from build123d import *

# Parameters (mm, degrees)
SKETCH1_R           = 50
SKETCH1_R_2         = 4
BOSS_EXTRUDE1_DEPTH = 10
BOSS_EXTRUDE2_START = 50
SKETCH2_R           = 50
SKETCH2_R_2         = 40
BOSS_EXTRUDE2_DEPTH = 50
BOSS_EXTRUDE3_START = 10
SKETCH4_R           = 4
SKETCH4_R_2         = 40
BOSS_EXTRUDE3_DEPTH = 10


with BuildPart() as part:
    # Sketch1 → Boss-Extrude1 (new body)
    with BuildSketch(Plane(origin=(0, 0, 0), x_dir=(1, 0, 0), z_dir=(0, 1, 0))):
        with Locations(Location((0, 0, 0), (0, 0, 270))):
            Circle(SKETCH1_R)
        with Locations(Location((0, 0, 0), (0, 0, 270))):
            Circle(SKETCH1_R_2, mode=Mode.SUBTRACT)
    extrude(amount=BOSS_EXTRUDE1_DEPTH)

    # Sketch2 → Boss-Extrude2 (add)
    with BuildSketch(Plane.XZ.offset(BOSS_EXTRUDE2_START)):
        with Locations(Location((0, 0, 0), (0, 0, 270))):
            Circle(SKETCH2_R)
        with Locations(Location((0, 0, 0), (0, 0, 270))):
            Circle(SKETCH2_R_2, mode=Mode.SUBTRACT)
    extrude(amount=-BOSS_EXTRUDE2_DEPTH)

    # Sketch4 → Boss-Extrude3 (add)
    with BuildSketch(Plane.XZ.offset(50).offset(BOSS_EXTRUDE3_START)):
        with BuildLine():
            Line((-30.18665216, -50), (29.99743133, -50))
            Line((29.99743133, -50), (45.000642085, -58.660624714))
            ThreePointArc((45.000642085, -58.660624714), (57.090562914, -57.051518812), (58.632887989, -44.95289737))
            Line((58.632887989, -44.95289737), (50, -30.18665216))
            Line((50, -30.18665216), (50, 29.99743133))
            Line((50, 29.99743133), (58.660624714, 45.000642085))
            ThreePointArc((58.660624714, 45.000642085), (57.051518812, 57.090562914), (44.95289737, 58.632887989))
            Line((44.95289737, 58.632887989), (30.18665216, 50))
            Line((30.18665216, 50), (-29.99743133, 50))
            Line((-29.99743133, 50), (-45.000642085, 58.660624714))
            ThreePointArc((-45.000642085, 58.660624714), (-57.090562914, 57.051518812), (-58.632887989, 44.95289737))
            Line((-58.632887989, 44.95289737), (-50, 30.18665216))
            Line((-50, 30.18665216), (-50, -29.99743133))
            Line((-50, -29.99743133), (-58.660624714, -45.000642085))
            ThreePointArc((-58.660624714, -45.000642085), (-57.051518812, -57.090562914), (-44.95289737, -58.632887989))
            Line((-44.95289737, -58.632887989), (-30.18665216, -50))
        make_face()
        with Locations(Location((-50, 50, 0), (0, 0, 270))):
            Circle(SKETCH4_R, mode=Mode.SUBTRACT)
        with Locations(Location((-50, -50, 0), (0, 0, 270))):
            Circle(SKETCH4_R, mode=Mode.SUBTRACT)
        with Locations(Location((50, -50, 0), (0, 0, 90))):
            Circle(SKETCH4_R, mode=Mode.SUBTRACT)
        with Locations(Location((50, 50, 0), (0, 0, 90))):
            Circle(SKETCH4_R, mode=Mode.SUBTRACT)
        with Locations(Location((0, 0, 0), (0, 0, 270))):
            Circle(SKETCH4_R_2, mode=Mode.SUBTRACT)
    extrude(amount=-BOSS_EXTRUDE3_DEPTH)


solid = part.part
The listing builds one solid part. Answer for the finished solid, in the listing's coordinates (mm). A direction names the side the tool comes from. Give positions to 0.01 mm unless a question says otherwise; leave off trailing zeros. Write each loop counter-clockwise with the first axis right and the second up, starting at its lowest first coordinate (ties: lowest second). Pieces come first, ordered by that corner, then holes. Notation, with made-up numbers: (-29, -26.75) -> (4, -26.75) arc R17 ccw to (4, -0.75) -> close; hole circle Ø11 at (55.5, 12). An arc over 180 degrees is marked (long way). Use a Markdown table: item, result.
(1) Section D-D, the plane z = 48 is taken. Determine the outline of the cut face in (x, y).
Return value:
| item | result |
|---|---|
| outline | (-59.8, -60) -> (-53.46, -60) -> (-53.46, -50) -> (-59.8, -50) -> close; (-46.54, -60) -> (46.54, -60) -> (46.54, -50) -> (14, -50) -> (14, 10) -> (-14, 10) -> (-14, -50) -> (-46.54, -50) -> close; (53.46, -60) -> (59.8, -60) -> (59.8, -50) -> (53.46, -50) -> close |
(2) Section A-A, the plane y = -1.5 is taken. Determine the outline of the cut face in (x, z).
Return value:
| item | result |
|---|---|
| outline | circle Ø100 at (0, 0); hole circle Ø80 at (0, 0) |
(3) For faces 4 (the flat face through (54.27, -55.07, 37.394)), 5 (the flat face through (1, 0, 8)), 6 (the flat face through (-50, -55, 1)), 7 (the flat face through (-37.394, -55.07, 54.27)), 8 (the flat face through (-1, -55, -50)), determine the directions among +Z, -Z, +X, -X, +Y, -Y from which every point of the face is accessible in a straight line to the end or side of a thin tool.
Return value:
| item | result |
|---|---|
| face 4 | +X, +Y, -Y |
| face 5 | -Y |
| face 6 | -X, +Y, -Y |
| face 7 | +Z, +Y, -Y |
| face 8 | -Z, +Y, -Y |
(4) Determine the mould class of faces 1 (the flat face through (37.673, -55.07, 54.377)), 2 (the cylindrical face through (-52.4, -55.1, 53.2)), 3 (the flat face through (-41, -50, 43)) for opening direction Z: released by +Z, released by -Z, zero draft, split by the parting line, or undercut.
Return value:
| item | result |
|---|---|
| face 1 | released by +Z |
| face 2 | undercut |
| face 3 | zero draft |
(5) Section B-B, the plane z = -42.5 is taken. Determine the outline of the cut face in (x, y), then the cut area to 3 significant figures.
Return value:
| item | result |
|---|---|
| outline | (-57.22, -60) -> (57.2, -60) -> (57.2, -50) -> (26.34, -50) -> (26.34, 10) -> (-26.34, 10) -> (-26.34, -50) -> (-57.22, -50) -> close |
| area | 4,300 mm2 |
(6) Flat-ended cylindrical pins translate along their axes: P1, Ø7, axis at x = -50, z = -50, coming from the +Y side; P2, Ø8, axis at x = -6, y = -52, coming from the +Z side; P3, Ø3, axis at x = 32, z = -17.5, coming from the -Y side; P4, Ø10.5, axis at x = 50, z = -50, coming from the +Y side. Find the tip coordinate at first contact, or state that the pin passes through.
Return value:
| item | result |
|---|---|
| P1 | through |
| P2 | z = 50 |
| P3 | y = 0 |
| P4 | y = -50 |
(7) Find the intervals of material crossed by probe 1 along X at (y, z) = (5.5, 0); probe 2 along X at (y, z) = (-17.5, 0.5); probe 3 along Z at (x, y) = (-15, -13.5), in increasing order. Write a range as from..to.
Return value:
| item | result |
|---|---|
| probe 1 | -50..-4, 4..50 |
| probe 2 | -50..-40, 40..50 |
| probe 3 | -47.7..-37.08, 37.08..47.7 |
(8) Section C-C, the plane x = -9.5 is taken. Determine the outline of the cut face in (y, z), then the cut area to 3 significant figures.
Return value:
| item | result |
|---|---|
| outline | (-60, -50) -> (-50, -50) -> (-50, -49.09) -> (10, -49.09) -> (10, 49.09) -> (-50, 49.09) -> (-50, 50) -> (-60, 50) -> (-60, 38.86) -> (0, 38.86) -> (0, -38.86) -> (-60, -38.86) -> close |
| area | 2,230 mm2 |
